Check sheet for the modelled part. Datum: model origin and axes. Units: mm. Coordinates: 2 decimals unless noted, no trailing zeros. Order: outer loops, then holes, each group sorted by start corner. A loop starts at its lowest first (then second) coordinate and runs counter-clockwise, first axis right, second up.
from build123d import *

# Parameters (mm, degrees)
F0_W     = 50.8
F0_H     = 914.4
F1_DEPTH = 50.8
F2_D     = 25.4


with BuildPart() as f1:
    # F0 (on Right) → F1 (new body)
    with BuildSketch(Plane.YZ):
        Rectangle(F0_W, F0_H)
    extrude(amount=F1_DEPTH)

    # F2 (through all)
    with Locations(Plane(origin=(0, 0, 0), x_dir=(0, 1, 0), z_dir=(-1, 0, 0))):
        with Locations((0, 406.4), (0, -406.4)):
            Hole(F2_D / 2)


solid = f1.part
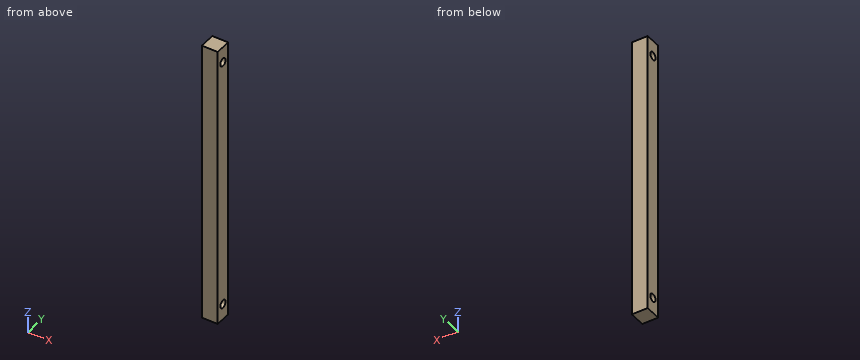
(1) Cross-section at B-B (z = -406.4). Enter the section's corners in (x, y), and give its area (3 significant figures).
Filled in:
outline: (0, -25.4) - (50.8, -25.4) - (50.8, -12.7) - (0, -12.7) - close; (0, 12.7) - (50.8, 12.7) - (50.8, 25.4) - (0, 25.4) - close
area: 1,290 mm2
(2) Cross-section at C-C (x = 43). Enter the section's corners in (y, z), and give its area (3 significant figures).
Filled in:
outline: (-25.4, -457.2) - (25.4, -457.2) - (25.4, 457.2) - (-25.4, 457.2) - close; hole circle Ø25.4 at (0, -406.4); hole circle Ø25.4 at (0, 406.4)
area: 45,400 mm2
(3) Cross-section at A-A (y = 0). Enter the section's corners in (x, z).
Filled in:
outline: (0, -457.2) - (50.8, -457.2) - (50.8, -419.1) - (0, -419.1) - close; (0, -393.7) - (50.8, -393.7) - (50.8, 393.7) - (0, 393.7) - close; (0, 419.1) - (50.8, 419.1) - (50.8, 457.2) - (0, 457.2) - close
(4) Thickness scan on probe 1 along Z at (x, y) = (34, 0); probe 2 along Z at (x, y) = (42.5, -5); probe 3 along Y at (x, z) = (37, -406). Record the ranges inside material, lowest first.
Filled in:
probe 1: z = -457.2 to -419.1, -393.7 to 393.7, 419.1 to 457.2
probe 2: z = -457.2 to -418.07, -394.73 to 394.73, 418.07 to 457.2
probe 3: y = -25.4 to -12.69, 12.69 to 25.4
